For this review, take the finished solid that the model builds, in its own axes (mm). A direction names the side the tool comes from. Coordinates: 2 decimals unless noted, no trailing zeros. Order: outer loops, then holes, each group sorted by start corner. A loop starts at its lowest first (then second) coordinate and runs counter-clockwise, first axis right, second up. Notation, with made-up numbers: (75, 16) - (96, 16) arc R15 ccw to (96, 35) - close; hole circle Ø5 at (-13, 70). An arc over 180 degrees is marked (long way). One line per item, written item: value. Start each with the question number.
(1) Mouldability with a two-part tool opening along Z and no side actions: class faces 5 (the cylindrical face through (8, 4, -10)), 6 (the cylindrical face through (0.86, 4.06, -24.1)), 7 (the cylindrical face through (11.22, 3.94, 7.71)) as released by +Z, released by -Z, zero draft, split by the parting line, or undercut.
(2) For faces 1 (the flat face through (6.5, 4.1, 1.6)), 2 (the flat face through (4, 4, 0)), 3 (the flat face through (12, 4, 0)), 4 (the cylindrical face through (15.1, 4.06, -24.14)), list the 3-axis set-ups (+Z, -Z, +X, -X, +Y, -Y) from which the entire face can be reached by the end or side of a thin tool; tool diameter is ignored.
(3) Consider section B-B on z = 1.5. Write out the cut boundary in (x, y), then the cut area to 3 significant figures.
(4) Consider section D-D on z = -6. Write out the cut boundary in (x, y), then the cut area to 3 significant figures.
(5) Clearance check with flat-ended pins moving along their axes: pin 1 (5 mm diameter, centred on x = 8, z = -6, fed in from -Y); pin 2 (0.8 mm diameter, centred on x = 4, y = 5, fed in from +Z); pin 3 (4 mm diameter, centred on y = 5.5, z = 1, fed in from +X); pin 4 (2.5 mm diameter, centred on y = 3, z = -1, fed in from -X). State where each tip first meets the part, or that it passes through.
(6) Consider section A-A on y = 4. Count the separate pieces of the cut face and the enclosed holes in it, then the cut area to 3 significant figures.
(7) To check wall thickness, follow line 1 along X through (y, z) = (6.5, -21); line 2 along Z through (x, y) = (10.5, 4.25); line 3 along Y through (x, z) = (10, 3.5). State the ranges of each line that lie inside material, in increasing order.
```python
from build123d import *

# Parameters (mm, degrees)
SKETCH1_W           = 16
SKETCH1_H           = 25
SKETCH1_R           = 1.45
SKETCH1_R_2         = 4
BOSS_EXTRUDE1_DEPTH = 8
FILLET1_R           = 3
SKETCH2_W           = 2
SKETCH2_H           = 8
BOSS_EXTRUDE2_DEPTH = 8
FILLET2_R           = 1
FILLET3_R           = 1
CUT_EXTRUDE1_DEPTH  = 31.740852298
SKETCH5_R           = 1.45
CUT_EXTRUDE3_DEPTH  = 29.664809327


with BuildPart() as part:
    # Sketch1 → Boss-Extrude1 (new body)
    with BuildSketch(Plane(origin=(0, 0, 0), x_dir=(1, 0, 0), z_dir=(0, 1, 0))):
        with Locations((8, 12.5)):
            Rectangle(SKETCH1_W, SKETCH1_H)
        with Locations(Location((8, 21, 0), (0, 0, 270))):
            Circle(SKETCH1_R, mode=Mode.SUBTRACT)
        with Locations(Location((8, 6, 0), (0, 0, 270))):
            Circle(SKETCH1_R_2, mode=Mode.SUBTRACT)
    extrude(amount=BOSS_EXTRUDE1_DEPTH)

    # Fillet1
    fillet1_edges = [part.edges().sort_by_distance(p)[0] for p in [
        (0, 4, -25),
        (16, 4, -25),
        (16, 4, 0),
        (0, 4, 0),
    ]]
    fillet(fillet1_edges, radius=FILLET1_R)

    # Sketch2 → Boss-Extrude2 (add, through all)
    with BuildSketch(Plane(origin=(0, 8, 0), x_dir=(1, 0, 0), z_dir=(0, 1, 0))):
        with Locations((5.5, -4)):
            Rectangle(SKETCH2_W, SKETCH2_H)
        with Locations((10.518302555, -4)):
            Rectangle(SKETCH2_W, SKETCH2_H)
    extrude(amount=-BOSS_EXTRUDE2_DEPTH)

    # Fillet2
    fillet2_edges = [part.edges().sort_by_distance(p)[0] for p in [
        (4.5, 4, 8),
    ]]
    fillet(fillet2_edges, radius=FILLET2_R)

    # Fillet3
    fillet3_edges = [part.edges().sort_by_distance(p)[0] for p in [
        (11.518302555, 4, 8),
    ]]
    fillet(fillet3_edges, radius=FILLET3_R)

    # Sketch3 → Cut-Extrude1 (cut, through all)
    with BuildSketch(Plane(origin=(0, 8, 0), x_dir=(1, 0, 0), z_dir=(0, 1, 0))):
        with BuildLine():
            Line((6.5, 2.291900756), (6.5, -1.76134076))
            Line((6.5, -1.76134076), (9.493627756, -1.76134076))
            Line((9.493627756, -1.76134076), (9.493627756, 2.289329423))
            ThreePointArc((9.493627756, 2.289329423), (7.996564259, 2.000001476), (6.5, 2.291900756))
        make_face()
    extrude(amount=-CUT_EXTRUDE1_DEPTH, mode=Mode.SUBTRACT)

    # Sketch5 → Cut-Extrude3 (cut, through all)
    with BuildSketch(Plane(origin=(11.518302555, 0, 0), x_dir=(0, 0, -1), z_dir=(1, 0, 0))):
        with Locations((-3.5, 4)):
            Circle(SKETCH5_R)
    extrude(amount=-CUT_EXTRUDE3_DEPTH, mode=Mode.SUBTRACT)


solid = part.part
```
Geometry check:
1. face 5: undercut
1. face 6: released by -Z
1. face 7: released by +Z
2. face 1: +Z, +Y, -Y
2. face 2: +Z, -X, +Y, -Y
2. face 3: +Z, +X, +Y, -Y
2. face 4: -Z, +X, +Y, -Y
3. outline: (4.5, 0) - (6.5, 0) - (6.5, 8) - (4.5, 8) - close; (9.52, 0) - (11.52, 0) - (11.52, 8) - (9.52, 8) - close
3. area: 32.0 mm^2
4. outline: (0, 0) - (4, 0) - (4, 8) - (0, 8) - close; (12, 0) - (16, 0) - (16, 8) - (12, 8) - close
4. area: 64.0 mm^2
5. pin 1: passes through
5. pin 2: stops at z = 0
5. pin 3: stops at x = 15.24
5. pin 4: stops at x = 0.1
6. separate pieces: 3
6. enclosed holes: 1
6. area: 349 mm^2
7. line 1: x = 0 to 6.55, 9.45 to 16
7. line 2: z = -25 to -9.12, -2.88 to 2.07, 4.93 to 8
7. line 3: y = 0 to 2.55, 5.45 to 8
